```python
from build123d import *

# Parameters (mm, degrees)
F0_R     = 4.6
F1_DEPTH = 10
F0_R_2   = 2.5
F2_DEPTH = 3


# Not quite as in the source:
# - ends of sketch curves that miss each other by under 0.0002 mm in the source are joined


with BuildPart() as f1:
    # F0 (on Top) → F1 (new body)
    with BuildSketch(Plane.XY):
        with BuildLine():
            ThreePointArc((-40, -61), (-39.5606601718, -62.0606601718), (-38.5, -62.5))
            Line((-38.5, -62.5), (35, -62.5))
            ThreePointArc((35, -62.5), (38.5355339059, -61.0355339059), (40, -57.5))
            Line((40, -57.5), (40, -47.5))
            ThreePointArc((40, -47.5), (38.5355339059, -43.9644660941), (35, -42.5))
            Line((35, -42.5), (14.571067, -42.5))
            ThreePointArc((14.571067, -42.5), (12.6576501648, -42.1193977979), (11.0355335941, -41.0355344059))
            Line((11.0355335941, -41.0355344059), (1.464466, -31.464466))
            ThreePointArc((1.464466, -31.464466), (0.3806023374, -29.8423491618), (0, -27.928932))
            Line((0, -27.928932), (0, -17.071068))
            ThreePointArc((0, -17.071068), (0.3806023374, -15.1576508382), (1.4644660941, -13.5355340941))
            Line((1.4644660941, -13.5355340941), (11.035534, -3.964466))
            ThreePointArc((11.035534, -3.964466), (12.6576501648, -2.8806022021), (14.571067, -2.5))
            Line((14.571067, -2.5), (35, -2.5))
            ThreePointArc((35, -2.5), (38.5355339059, -1.0355339059), (40, 2.5))
            Line((40, 2.5), (40, 12.5))
            ThreePointArc((40, 12.5), (38.5355339059, 16.0355339059), (35, 17.5))
            Line((35, 17.5), (0.62132, 17.5))
            ThreePointArc((0.62132, 17.5), (0.0472948515, 17.6141807012), (-0.4393401718, 17.9393398282))
            Line((-0.4393401718, 17.9393398282), (-19.560661, 37.06066))
            ThreePointArc((-19.560661, 37.06066), (-19.8858192988, 37.5472958515), (-20, 38.121321))
            Line((-20, 38.121321), (-20, 61))
            ThreePointArc((-20, 61), (-20.4393398282, 62.0606601718), (-21.5, 62.5))
            Line((-21.5, 62.5), (-38.5, 62.5))
            ThreePointArc((-38.5, 62.5), (-39.5606601718, 62.0606601718), (-40, 61))
            Line((-40, 61), (-40, -61))
        make_face()
        with Locations((-30, -52.5)):
            Circle(F0_R, mode=Mode.SUBTRACT)
        with Locations((-10, -32.5)):
            Circle(F0_R, mode=Mode.SUBTRACT)
        with Locations((-10, -12.5)):
            Circle(F0_R, mode=Mode.SUBTRACT)
        with Locations((10, -52.5)):
            Circle(F0_R, mode=Mode.SUBTRACT)
        with Locations((30, -52.5)):
            Circle(F0_R, mode=Mode.SUBTRACT)
        with Locations((-30, 7.5)):
            Circle(F0_R, mode=Mode.SUBTRACT)
        with Locations((-30, 47.5)):
            Circle(F0_R, mode=Mode.SUBTRACT)
        with BuildLine():
            Line((-36, 54.53), (-36, 56.65))
            ThreePointArc((-36, 56.65), (-35.5782337649, 57.6682337649), (-34.56, 58.09))
            Line((-34.56, 58.09), (-25.44, 58.09))
            ThreePointArc((-25.44, 58.09), (-24.4217662351, 57.6682337649), (-24, 56.65))
            Line((-24, 56.65), (-24, 54.53))
            ThreePointArc((-24, 54.53), (-24.4217662351, 53.5117662351), (-25.44, 53.09))
            Line((-25.44, 53.09), (-34.56, 53.09))
            ThreePointArc((-34.56, 53.09), (-35.5782337649, 53.5117662351), (-36, 54.53))
        make_face(mode=Mode.SUBTRACT)
        with Locations((10, 7.5)):
            Circle(F0_R, mode=Mode.SUBTRACT)
        with Locations((30, 7.5)):
            Circle(F0_R, mode=Mode.SUBTRACT)
    extrude(amount=F1_DEPTH)

    # F0 (on Top) → F2 (join)
    with BuildSketch(Plane.XY):
        with Locations((-30, 47.5)):
            Circle(F0_R)
        with Locations((-30, 47.5)):
            Circle(F0_R_2, mode=Mode.SUBTRACT)
        with Locations((-30, 7.5)):
            Circle(F0_R)
        with Locations((-30, 7.5)):
            Circle(F0_R_2, mode=Mode.SUBTRACT)
        with Locations((-30, -52.5)):
            Circle(F0_R)
        with Locations((-30, -52.5)):
            Circle(F0_R_2, mode=Mode.SUBTRACT)
        with Locations((-10, -32.5)):
            Circle(F0_R)
        with Locations((-10, -32.5)):
            Circle(F0_R_2, mode=Mode.SUBTRACT)
        with Locations((10, -52.5)):
            Circle(F0_R)
        with Locations((10, -52.5)):
            Circle(F0_R_2, mode=Mode.SUBTRACT)
        with Locations((30, -52.5)):
            Circle(F0_R)
        with Locations((30, -52.5)):
            Circle(F0_R_2, mode=Mode.SUBTRACT)
        with Locations((-10, -12.5)):
            Circle(F0_R)
        with Locations((-10, -12.5)):
            Circle(F0_R_2, mode=Mode.SUBTRACT)
        with Locations((10, 7.5)):
            Circle(F0_R)
        with Locations((10, 7.5)):
            Circle(F0_R_2, mode=Mode.SUBTRACT)
        with Locations((30, 7.5)):
            Circle(F0_R)
        with Locations((30, 7.5)):
            Circle(F0_R_2, mode=Mode.SUBTRACT)
    extrude(amount=F2_DEPTH)


solid = f1.part
```
Can you work these out from the model? Positions are in its coordinate system, mm. A direction names the side the tool comes from. Give positions to 0.01 mm unless a question says otherwise; leave off trailing zeros. Order: outer loops, then holes, each group sorted by start corner. A loop starts at its lowest first (then second) coordinate and runs counter-clockwise, first axis right, second up. Notation, with made-up numbers: (69.25, 39.25) - (125.25, 39.25) arc R14 cw to (125.25, 47.25) - close; hole circle Ø11 at (59.5, 73.25). An arc over 180 degrees is marked (long way). Use a Markdown table: item, result. Add a question column.
Q1. If we section it at D-D on z = 5: Count the separate pieces of the cut face and the enclosed holes in it, plus the area to 3 significant figures.
Q2. If we section it at B-B on x = -10: Write out the boundary of the cut face in (y, z).
Q3. If we section it at C-C on x = 30: Write out the boundary of the cut face in (y, z).
Q4. If we section it at A-A on y = -52.5: Write out the boundary of the cut face in (x, z), plus the area to 3 significant figures.
Q5. If we mould it in two halves opening along Y, with no side actions, what happens to faces 1 (the flat face through (12, -54.5, 3)), 2 (the cylindrical face through (38.57, 16, 4.93)), 3 (the flat face through (40, -53, 5))? For each: released by +Y, released by -Y, zero draft, split by the parting line, or undercut.
Q6. Please list where these lines run through material, in increasing order: line 1 along Y through (x, z) = (-30, 7.25); line 2 along Y through (x, z) = (-10, 6); line 3 along Y through (x, z) = (30, 1.5).
Q7. I'm going to push flat-ended pins straight in: pin 1 (4 mm diameter, centred on x = -30, y = 7.5, fed in from +Z); pin 2 (3 mm diameter, centred on x = 31, y = -53, fed in from +Z); pin 3 (3 mm diameter, centred on y = 47, z = 4.5, fed in from +X); pin 4 (4 mm diameter, centred on y = -16.5, z = 2.5, fed in from +X). Where does each tip first touch, or does it pass through?
Q8. On a 3-axis mill with a long thin cutter (end or side, diameter ignored), from which of +Z, -Z, +X, -X, +Y, -Y can I reach the whole of each face in a straight line? I mean faces 4 (the cylindrical face through (-27.877, 43.419, 6.451)), 5 (the cylindrical face through (12.68, -42.13, 4.93)), 6 (the flat face through (-18, -13, 10)), 7 (the cylindrical face through (29.46, -54.94, 1.48)), 8 (the flat face through (18, 17.5, 5)). Say none if no direction works.
Answers follow:
| question | item | result |
|---|---|---|
| 1 | separate pieces | 1 |
| 1 | enclosed holes | 10 |
| 1 | area | 5,380 mm^2 |
| 2 | outline | (-62.5, 0) - (-35, 0) - (-35, 3) - (-37.1, 3) - (-37.1, 10) - (-62.5, 10) - close; (-30, 0) - (-15, 0) - (-15, 3) - (-17.1, 3) - (-17.1, 10) - (-27.9, 10) - (-27.9, 3) - (-30, 3) - close; (-10, 0) - (27.5, 0) - (27.5, 10) - (-7.9, 10) - (-7.9, 3) - (-10, 3) - close |
| 3 | outline | (-62.5, 0) - (-55, 0) - (-55, 3) - (-57.1, 3) - (-57.1, 10) - (-62.5, 10) - close; (-50, 0) - (-42.5, 0) - (-42.5, 10) - (-47.9, 10) - (-47.9, 3) - (-50, 3) - close; (-2.5, 0) - (5, 0) - (5, 3) - (2.9, 3) - (2.9, 10) - (-2.5, 10) - close; (10, 0) - (17.5, 0) - (17.5, 10) - (12.1, 10) - (12.1, 3) - (10, 3) - close |
| 4 | outline | (-40, 0) - (-32.5, 0) - (-32.5, 3) - (-34.6, 3) - (-34.6, 10) - (-40, 10) - close; (-27.5, 0) - (7.5, 0) - (7.5, 3) - (5.4, 3) - (5.4, 10) - (-25.4, 10) - (-25.4, 3) - (-27.5, 3) - close; (12.5, 0) - (27.5, 0) - (27.5, 3) - (25.4, 3) - (25.4, 10) - (14.6, 10) - (14.6, 3) - (12.5, 3) - close; (32.5, 0) - (40, 0) - (40, 10) - (34.6, 10) - (34.6, 3) - (32.5, 3) - close |
| 4 | area | 562 mm^2 |
| 5 | face 1 | undercut |
| 5 | face 2 | released by +Y |
| 5 | face 3 | zero draft |
| 6 | line 1 | y = -62.5 to -57.1, -47.9 to 2.9, 12.1 to 42.9, 52.1 to 53.09, 58.09 to 62.5 |
| 6 | line 2 | y = -62.5 to -37.1, -27.9 to -17.1, -7.9 to 27.5 |
| 6 | line 3 | y = -62.5 to -55, -50 to -42.5, -2.5 to 5, 10 to 17.5 |
| 7 | pin 1 | passes through |
| 7 | pin 2 | stops at z = 3 |
| 7 | pin 3 | stops at x = -20 |
| 7 | pin 4 | stops at x = 0.71 |
| 8 | face 4 | +Z |
| 8 | face 5 | +Z, -Z, +X |
| 8 | face 6 | +Z, +X, -X, +Y, -Y |
| 8 | face 7 | +Z, -Z |
| 8 | face 8 | +Z, -Z, +X, +Y |
